The listing builds one solid part. Answer for the finished solid, in the listing's coordinates (mm). Round coordinates to 2 decimals unless told otherwise and drop trailing zeros. Loops run counter-clockwise (first coordinate to the right, second up) from the corner with the lowest first, then second, coordinate; pieces in that order, holes last. Notation, with made-up numbers: M 43.25,-3 L 58.25,-3 A27 cw 58.25,18 Z; hole C 82.25,-23 d3. An arc over 180 degrees is marked long. Put each result on its own line as item: value. Start each with the question number.
(1) Flat-ended cylindrical pins translate along their axes: P1, Ø1.5, axis at x = 2.5, z = 5.5, coming from the -Y side; P2, Ø3, axis at y = 2, z = 3, coming from the -X side; P3, Ø2, axis at x = -12, z = 1, coming from the -Y side. Find the tip coordinate at first contact, or state that the pin passes through.
(2) Section D-D, the plane y = 13 is taken. Determine the outline of the cut face in (x, z).
(3) Section B-B, the plane y = 0 is taken. Determine the outline of the cut face in (x, z) (3 decimals), then the cut area to 3 significant figures.
(4) Section A-A, the plane x = 0 is taken. Determine the outline of the cut face in (y, z).
(5) Straight lines are drawn through the part: line 1 (Y direction, x = 0, z = 3.5); line 2 (X direction, y = -13.5, z = 3.75); line 3 (X direction, y = 0.5, z = 0.75). For each, find the intervals that lie inside material, in ascending order.
(6) Section C-C, the plane z = 5.5 is taken. Count the separate pieces of the cut face and the enclosed holes in it, then the cut area to 3 significant figures.
(7) Determine the mould class of faces 1 (the face through (-17.143, 0.07, 3.131)), 2 (the face through (0, 0, 6.35)), 3 (the face through (-15.12, -11.59, 3.13)) for opening direction X: released by +X, released by -X, zero draft, split by the parting line, or undercut.
```python
from build123d import *

# Parameters (mm, degrees)
SKETCH1_R           = 19.05
SKETCH1_R_2         = 6.0325
SKETCH1_R_3         = 1.5875
BOSS_EXTRUDE1_DEPTH = 6.35


with BuildPart() as part:
    # Sketch1 → Boss-Extrude1 (new body)
    with BuildSketch(Plane.XY):
        Circle(SKETCH1_R)
        with Locations((0, -6.858)):
            Circle(SKETCH1_R_2, mode=Mode.SUBTRACT)
        with Locations((-7.77875, 13.473190219)):
            Circle(SKETCH1_R_3, mode=Mode.SUBTRACT)
        with Locations((7.77875, 13.473190219)):
            Circle(SKETCH1_R_3, mode=Mode.SUBTRACT)
        with Locations((15.5575, 0)):
            Circle(SKETCH1_R_3, mode=Mode.SUBTRACT)
        with Locations((7.77875, -13.473190219)):
            Circle(SKETCH1_R_3, mode=Mode.SUBTRACT)
        with Locations((-7.77875, -13.473190219)):
            Circle(SKETCH1_R_3, mode=Mode.SUBTRACT)
        with Locations((-15.5575, 0)):
            Circle(SKETCH1_R_3, mode=Mode.SUBTRACT)
    extrude(amount=BOSS_EXTRUDE1_DEPTH)


solid = part.part
```
Recorded:
1. P1: stops at y = -18.97
1. P2: stops at x = -19.04
1. P3: stops at y = -15.55
2. outline: M -13.92,0 L -9.29,0 L -9.29,6.35 L -13.92,6.35 Z; M -6.26,0 L 6.26,0 L 6.26,6.35 L -6.26,6.35 Z; M 9.29,0 L 13.92,0 L 13.92,6.35 L 9.29,6.35 Z
3. outline: M -19.05,0 L -17.145,0 L -17.145,6.35 L -19.05,6.35 Z; M -13.97,0 L 13.97,0 L 13.97,6.35 L -13.97,6.35 Z; M 17.145,0 L 19.05,0 L 19.05,6.35 L 17.145,6.35 Z
3. area: 202 mm²
4. outline: M -19.05,0 L -12.89,0 L -12.89,6.35 L -19.05,6.35 Z; M -0.83,0 L 19.05,0 L 19.05,6.35 L -0.83,6.35 Z
5. line 1: y = -19.05 to -12.89, -0.83 to 19.05
5. line 2: x = -13.44 to -9.37, -6.19 to 6.19, 9.37 to 13.44
5. line 3: x = -19.04 to -17.06, -14.05 to 14.05, 17.06 to 19.04
6. separate pieces: 1
6. enclosed holes: 7
6. area: 978 mm²
7. face 1: undercut
7. face 2: zero draft
7. face 3: split by the parting line
